Input: part model. Units: mm. Frame: model coordinates. Face numbers are marked on the shaded views. A direction names the side the tool comes from. Round coordinates to 2 decimals unless told otherwise and drop trailing zeros. Loops run counter-clockwise (first coordinate to the right, second up) from the corner with the lowest first, then second, coordinate; pieces in that order, holes last.
1) Section A-A, the plane z = -22. Return loops of the section in (x, y) (3 decimals).
2) Section B-B, the plane x = 3. Return loops of the section in (y, z) (3 decimals), and give its area (3 significant figures).
3) First-contact query: pin 1 (3 mm diameter, centred on y = 16.5, z = -4, fed in from -X); pin 2 (2.5 mm diameter, centred on x = 3, z = -22, fed in from +Y). Flat tips, straight axial feed; report the tip coordinate or a pass-through.
4) Section D-D, the plane y = 24.5. Return loops of the section in (x, z) (3 decimals), and give its area (3 significant figures).
5) Access query for the marked faces 4 and 5. Directions: +Z, -Z, +X, -X, +Y, -Y. A direction counts if a zero-diameter tool reaches every point of the face in a straight line with its end or side. Return the directions, or none.
6) Draft query along Z for the marked faces 1, 2 and 3. Return one class per face: pulls with the +Z half, pulls with the -Z half, needs draft (parallel to the pull), parting line crosses it, or undercut.
7) Section C-C, the plane z = -19. Return loops of the section in (x, y) (3 decimals), and give its area (3 significant figures).
8) Ray query, line 1 along Z through (x, y) = (3, 1.65); line 2 along X through (y, z) = (2, -22) (3 decimals); line 3 along X through (y, z) = (22.25, -15.5) (3 decimals). Return the intervals inside material, ascending.
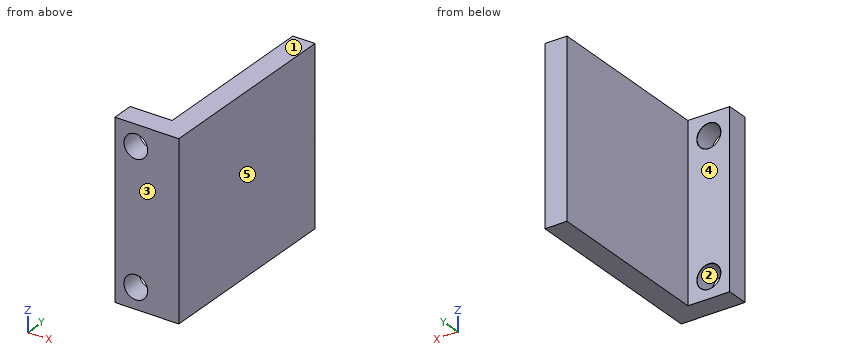
from build123d import *

# Parameters (mm, degrees)
SKETCH1_W                      = 9.175
SKETCH1_H                      = 25
BOSS_EXTRUDE1_DEPTH            = 3.175
SKETCH2_W                      = 3.175
SKETCH2_H                      = 25
BOSS_EXTRUDE2_DEPTH            = 25
M3_CLEARANCE_HOLE1_D           = 3.4
M3_CLEARANCE_HOLE1_CSINK_D     = 3.45
M3_CLEARANCE_HOLE1_CSINK_ANGLE = 90


with BuildPart() as part:
    # Sketch1 → Boss-Extrude1 (new body)
    with BuildSketch(Plane(origin=(0, 0, 0), x_dir=(1, 0, 0), z_dir=(0, 1, 0))):
        with Locations((4.5875, 12.5)):
            Rectangle(SKETCH1_W, SKETCH1_H)
    extrude(amount=BOSS_EXTRUDE1_DEPTH)

    # Sketch2 → Boss-Extrude2 (add)
    with BuildSketch(Plane(origin=(0, 3.175, 0), x_dir=(1, 0, 0), z_dir=(0, 1, 0))):
        with Locations((7.5875, 12.5)):
            Rectangle(SKETCH2_W, SKETCH2_H)
    extrude(amount=BOSS_EXTRUDE2_DEPTH)

    # M3 Clearance Hole1 (through all)
    with Locations(Plane(origin=(0, 3.175, 0), x_dir=(1, 0, 0), z_dir=(0, 1, 0))):
        with Locations((3, 22), (3, 3)):
            CounterSinkHole(M3_CLEARANCE_HOLE1_D / 2, M3_CLEARANCE_HOLE1_CSINK_D / 2, counter_sink_angle=M3_CLEARANCE_HOLE1_CSINK_ANGLE)


solid = part.part
Final values:
1. outline: (0, 0) - (1.3, 0) - (1.3, 3.15) - (1.275, 3.175) - (0, 3.175) - close; (4.7, 0) - (9.175, 0) - (9.175, 28.175) - (6, 28.175) - (6, 3.175) - (4.725, 3.175) - (4.7, 3.15) - close
2. outline: (0, -25) - (3.175, -25) - (3.175, -23.725) - (3.15, -23.7) - (0, -23.7) - close; (0, -20.3) - (3.15, -20.3) - (3.175, -20.275) - (3.175, -4.725) - (3.15, -4.7) - (0, -4.7) - close; (0, -1.3) - (3.15, -1.3) - (3.175, -1.275) - (3.175, 0) - (0, 0) - close
2. area: 57.8 mm2
3. pin 1: stops at x = 6
3. pin 2: passes through
4. outline: (6, -25) - (9.175, -25) - (9.175, 0) - (6, 0) - close
4. area: 79.4 mm2
5. face 4: +Z, -Z, -X, +Y
5. face 5: +Z, -Z, +X, +Y, -Y
6. face 1: pulls with the +Z half
6. face 2: undercut
6. face 3: needs draft
7. outline: (0, 0) - (9.175, 0) - (9.175, 28.175) - (6, 28.175) - (6, 3.175) - (0, 3.175) - close
7. area: 109 mm2
8. line 1: z = -25 to -23.7, -20.3 to -4.7, -1.3 to 0
8. line 2: x = 0 to 1.3, 4.7 to 9.175
8. line 3: x = 6 to 9.175
